```python
from build123d import *

# Parameters (mm, degrees)
SKETCH1_R                                       = 5
SKETCH1_R_2                                     = 1.6
SKETCH1_R_3                                     = 1.25
SKETCH1_R_4                                     = 1.55
BOSS_EXTRUDE1_DEPTH                             = 3.18
CHAMFER1_SIZE                                   = 5
CHAMFER1_SIZE2                                  = 0.881634904
CSK_FOR_M2_FLAT_HEAD_MACHINE_SCREW1_D           = 2.4
CSK_FOR_M2_FLAT_HEAD_MACHINE_SCREW1_DEPTH       = 3.508967257
CSK_FOR_M2_FLAT_HEAD_MACHINE_SCREW1_CSINK_D     = 4.4
CSK_FOR_M2_FLAT_HEAD_MACHINE_SCREW1_CSINK_ANGLE = 90
CSK_FOR_M2_FLAT_HEAD_MACHINE_SCREW1_TIP         = 0.721032743
SKETCH3_R                                       = 5
CUT_EXTRUDE4_DEPTH                              = 65.449891389
FILLET2_R                                       = 3
CHAMFER2_SIZE                                   = 1.8
FILLET4_R                                       = 0.5


with BuildPart() as part:
    # Sketch1 → Boss-Extrude1 (new body)
    with BuildSketch(Plane(origin=(0, 0, 0), x_dir=(0, 0, -1), z_dir=(1, 0, 0))):
        Polygon((0, 0), (0, 11.85), (7, 11.85), (7.5, 11.35), (8, 11.35), (8, 13.3), (0, 13.3), (0, 28.7), (2, 30.7), (2, 59.81), (22, 59.81), (22, 39.81), (23.8, 39.81), (23.8, 28.68), (14.1, 28.68), (14.1, 18.4), (11.85, 18.4), (11.85, 17), (23, 17), (23, 12), (12, 12), (12, 0), (8, 0), (8, 0.5), (7.5, 0.5), (7, 0), align=None)
        with Locations(Location((7, 23.7, 0), (0, 0, 180))):
            Circle(SKETCH1_R, mode=Mode.SUBTRACT)
        with Locations(Location((7, 55.31, 0), (0, 0, 180))):
            Circle(SKETCH1_R_2, mode=Mode.SUBTRACT)
        with Locations(Location((17, 53.31, 0), (0, 0, 180))):
            Circle(SKETCH1_R_2, mode=Mode.SUBTRACT)
        with Locations(Location((20.5, 14.5, 0), (0, 0, 180))):
            Circle(SKETCH1_R_3, mode=Mode.SUBTRACT)
        with Locations(Location((14.5, 14.5, 0), (0, 0, 180))):
            Circle(SKETCH1_R_3, mode=Mode.SUBTRACT)
        with Locations(Location((2.55, 2.55, 0), (0, 0, 180))):
            Circle(SKETCH1_R_4, mode=Mode.SUBTRACT)
        with Locations(Location((2.55, 8.55, 0), (0, 0, 180))):
            Circle(SKETCH1_R_4, mode=Mode.SUBTRACT)
    extrude(amount=BOSS_EXTRUDE1_DEPTH)

    # Chamfer1
    chamfer1_edges = [part.edges().sort_by_distance(p)[0] for p in [
        (1.59, 0, -12),
    ]]
    chamfer1_side = [part.faces().sort_by_distance(p)[0] for p in [
        (1.59, 6, -12),
    ]]
    chamfer(chamfer1_edges, length=CHAMFER1_SIZE, length2=CHAMFER1_SIZE2, reference=chamfer1_side[0])

    # CSK for M2 Flat Head Machine Screw1
    with Locations(Plane.ZY):
        with Locations((-6.974936087, 44.914674329), (-17.432559713, 40.744769284), (-8.592504199, 33.773154083)):
            CounterSinkHole(CSK_FOR_M2_FLAT_HEAD_MACHINE_SCREW1_D / 2, CSK_FOR_M2_FLAT_HEAD_MACHINE_SCREW1_CSINK_D / 2, depth=CSK_FOR_M2_FLAT_HEAD_MACHINE_SCREW1_DEPTH, counter_sink_angle=CSK_FOR_M2_FLAT_HEAD_MACHINE_SCREW1_CSINK_ANGLE)
            with Locations((0, 0, -(CSK_FOR_M2_FLAT_HEAD_MACHINE_SCREW1_DEPTH + CSK_FOR_M2_FLAT_HEAD_MACHINE_SCREW1_TIP / 2))):  # 118° drill point
                Cone(0, CSK_FOR_M2_FLAT_HEAD_MACHINE_SCREW1_D / 2, CSK_FOR_M2_FLAT_HEAD_MACHINE_SCREW1_TIP, mode=Mode.SUBTRACT)

    # Sketch3 → Cut-Extrude4 (cut, through all)
    with BuildSketch(Plane.ZY):
        with Locations((-11, 39.810865899)):
            Circle(SKETCH3_R)
    extrude(amount=-CUT_EXTRUDE4_DEPTH, mode=Mode.SUBTRACT)

    # Fillet2
    fillet2_edges = [part.edges().sort_by_distance(p)[0] for p in [
        (1.59, 28.7, 0),
        (1.59, 30.7, -2),
    ]]
    fillet(fillet2_edges, radius=FILLET2_R)

    # Chamfer2
    chamfer2_edges = [part.edges().sort_by_distance(p)[0] for p in [
        (1.59, 59.81, -22),
        (1.59, 59.81, -2),
        (1.59, 39.81, -23.8),
    ]]
    chamfer(chamfer2_edges, length=CHAMFER2_SIZE - 0.0001)  # a hair under: the kernel refuses the full size

    # Fillet4
    fillet4_edges = [part.edges().sort_by_distance(p)[0] for p in [
        (1.59, 0, -11.118365096),
        (1.59, 38.0101, -23.8),
        (1.59, 58.0101, -22),
        (1.59, 58.0101, -2),
        (1.59, 0, 0),
        (1.59, 11.85, 0),
        (1.59, 13.3, 0),
        (1.59, 18.4, -14.1),
    ]]
    fillet(fillet4_edges, radius=FILLET4_R)


solid = part.part
```
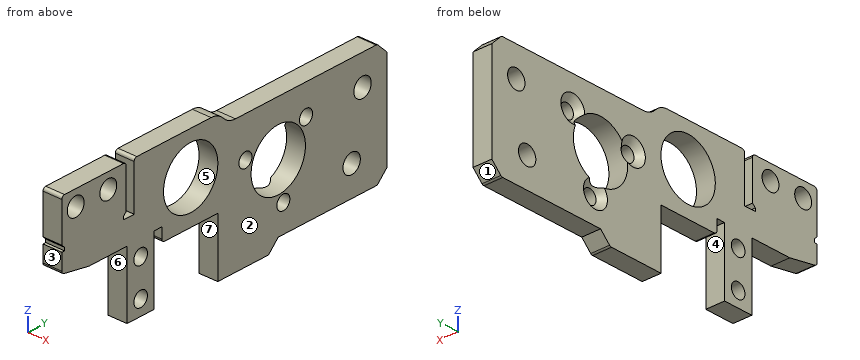
The listing builds one solid part. Answer for the finished solid, in the listing's coordinates (mm). Face numbers are marked on the shaded views. A direction names the side the tool comes from. Give positions to 0.01 mm unless a question says otherwise; leave off trailing zeros. Answer as a JSON object with one key per item and string values. Group by question number.
Item 1: A tool of negligible diameter and unlimited length cuts with its end or side. For the marked faces 5, 6 and 7, from which of +Z, -Z, +X, -X, +Y, -Y can it reach the whole face along a straight path? Write none if from no direction.
Item 2: Consider L1, parallel to Z at x = 1.85, y = 22.5; L2, parallel to Y at x = 1.85, z = -3; L3, parallel to Y at x = 1.6, z = -17. Determine where each line is inside the solid, lowest interval first. Write a range as from..to.
Item 3: Flat-ended cylindrical pins translate along their axes: pin 1 (4 mm diameter, centred on y = 40.74, z = -17.43, fed in from -X); pin 2 (1 mm diameter, centred on x = 2, z = -19, fed in from -Y); pin 3 (1.5 mm diameter, centred on x = 2.5, y = 18, fed in from -Z). Find the tip coordinate at first contact, or state that the pin passes through.
Item 4: Determine the mould class of the marked faces 1, 2, 3 and 4 for opening direction Y: pulls with the +Y half, pulls with the -Y half, needs draft (parallel to the pull), parting line crosses it, or undercut.
Item 5: The part is cut by section A-A on x = 1.85. Give the number of separate pieces and of enclosed holes in the cut face, and give its area (3 significant figures).
Result set:
{
 "1": {"face 5": "+X, -X", "face 6": "-Z, +X, -X, -Y", "face 7": "-Z, +X, -X"},
 "2": {"L1": "-14.1..-11.85, -2.15..0", "L2": "0..1.07, 4.03..7.07, 10.03..11.85, 13.3..20.7, 26.7..59.01", "L3": "12..17, 28.68..39.63, 41.86..51.71, 54.91..59.81"},
 "3": {"pin 1": "x = 0.19", "pin 2": "y = 12", "pin 3": "z = -14.08"},
 "4": {"face 1": "pulls with the +Y half", "face 2": "needs draft", "face 3": "pulls with the -Y half", "face 4": "undercut"},
 "5": {"separate pieces": "1", "enclosed holes": "11", "area": "834 mm²"}
}
